from build123d import *

# Parameters (mm, degrees)
BOSS_EXTRUDE1_DEPTH      = 10.6
BOSS_EXTRUDE1_DEPTH_BACK = 26.9
SKETCH1_W                = 40
SKETCH1_H                = 20
SKETCH1_3_W              = 40
SKETCH1_3_H              = 20
SKETCH1_3_W_2            = 7
SKETCH1_3_R              = 2
BOSS_EXTRUDE2_DEPTH      = 3
SKETCH2_R                = 3.307057182
BOSS_EXTRUDE3_DEPTH      = 1.5
BOSS_EXTRUDE4_START      = 1.5
SKETCH2_3_R              = 5.189986332
SKETCH2_3_R_2            = 3.307057182
BOSS_EXTRUDE4_DEPTH      = 6.5
FILLET1_R                = 3
FILLET2_R                = 1
BOSS_EXTRUDE6_DEPTH      = 1


with BuildPart() as part:
    # Sketch1 → Boss-Extrude1 (new, two sides: drawn at the far end of the back side and taken through both)
    with BuildSketch(Plane.XY.offset(-BOSS_EXTRUDE1_DEPTH_BACK)):
        Rectangle(SKETCH1_W, SKETCH1_H)
    extrude(amount=BOSS_EXTRUDE1_DEPTH + BOSS_EXTRUDE1_DEPTH_BACK)

    # Sketch1<3> → Boss-Extrude2 (add)
    # profile 1 of 3: a face of its own
    with BuildSketch(Plane.XY):
        Rectangle(SKETCH1_3_W, SKETCH1_3_H)
    # profile 2 of 3: a face of its own
    with BuildSketch(Plane.XY):
        with Locations((-23.5, 0)):
            Rectangle(SKETCH1_3_W_2, SKETCH1_3_H)
        with Locations((-24.3, -4.95)):
            Circle(SKETCH1_3_R, mode=Mode.SUBTRACT)
        with Locations((-24.3, 4.95)):
            Circle(SKETCH1_3_R, mode=Mode.SUBTRACT)
    # profile 3 of 3: a face of its own
    with BuildSketch(Plane.XY):
        with Locations((23.5, 0)):
            Rectangle(SKETCH1_3_W_2, SKETCH1_3_H)
        with Locations((24.3, -4.95)):
            Circle(SKETCH1_3_R, mode=Mode.SUBTRACT)
        with Locations((24.3, 4.95)):
            Circle(SKETCH1_3_R, mode=Mode.SUBTRACT)
    extrude(amount=BOSS_EXTRUDE2_DEPTH)

    # Sketch2 → Boss-Extrude3 (add)
    with BuildSketch(Plane.XY.offset(10.6)):
        with Locations((10, 0)):
            Circle(SKETCH2_R)
    extrude(amount=BOSS_EXTRUDE3_DEPTH)

    # Sketch2<3> → Boss-Extrude4 (add)
    # profile 1 of 2: a face of its own
    with BuildSketch(Plane.XY.offset(10.6).offset(BOSS_EXTRUDE4_START)):
        with Locations(Location((10, 0, 0), (0, 0, 180))):
            Circle(SKETCH2_3_R)
        with Locations((10, 0)):
            Circle(SKETCH2_3_R_2, mode=Mode.SUBTRACT)
    # profile 2 of 2: a face of its own
    with BuildSketch(Plane.XY.offset(10.6).offset(BOSS_EXTRUDE4_START)):
        with Locations((10, 0)):
            Circle(SKETCH2_3_R_2)
    extrude(amount=BOSS_EXTRUDE4_DEPTH)

    # Fillet1
    fillet1_edges = [part.edges().sort_by_distance(p)[0] for p in [
        (-27, 10, 1.5),
        (-27, -10, 1.5),
        (27, -10, 1.5),
        (27, 10, 1.5),
    ]]
    fillet(fillet1_edges, radius=FILLET1_R)

    # Fillet2
    fillet2_edges = [part.edges().sort_by_distance(p)[0] for p in [
        (20, 0, -26.9),
        (0, 10, 10.6),
        (-20, 0, 10.6),
        (0, -10, 10.6),
        (20, 0, 10.6),
        (0, 10, -26.9),
        (-20, 0, -26.9),
        (-20, -10, 6.8),
        (-20, 10, 6.8),
        (20, 10, 6.8),
        (0, -10, -26.9),
        (-20, -10, -13.45),
        (-20, 10, -13.45),
        (20, 10, -13.45),
        (20, -10, -13.45),
    ]]
    fillet(fillet2_edges, radius=FILLET2_R)

    # Sketch4 → Boss-Extrude6 (add, symmetric)
    with BuildSketch(Plane(origin=(0, 0, 0), x_dir=(1, 0, 0), z_dir=(0, 1, 0))):
        Polygon((-27, -3), (-20, -5.826634937), (-20, -3), align=None)
    boss_extrude6 = extrude(amount=BOSS_EXTRUDE6_DEPTH, both=True)

    # Mirror1: Boss-Extrude6 across plane
    add(boss_extrude6.mirror(Plane(origin=(0, 0, 0), x_dir=(0, 0, 1), z_dir=(1, 0, 0))))


solid = part.part
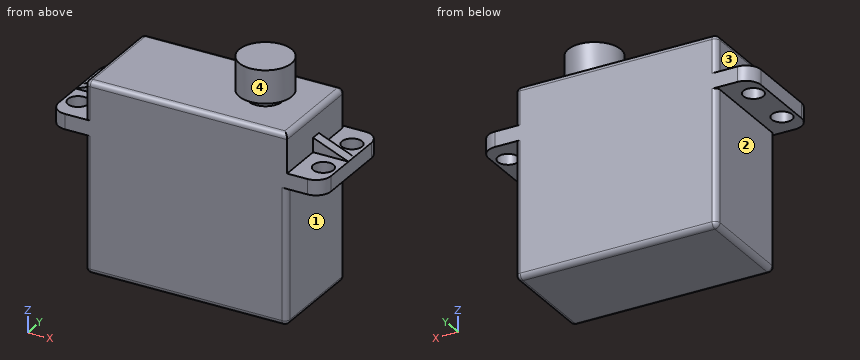
Model file for the job. Use its own axes, mm. Face numbers are marked on the shaded views. A direction names the side the tool comes from. Give positions to 0.01 mm unless a question says otherwise; leave off trailing zeros. Loops run counter-clockwise (first coordinate to the right, second up) from the corner with the lowest first, then second, coordinate; pieces in that order, holes last. Notation, with made-up numbers: (38.25, 68.5) - (75.25, 68.5) arc R24 ccw to (75.25, 102.5) - close; hole circle Ø5 at (30, 18). An arc over 180 degrees is marked (long way). Use one line per item in the form item = value.
(1) Drop flat-ended pins along their axis: P1, Ø3, axis at y = 6, z = -10, coming from the +X side; P2, Ø1, axis at x = 21, y = 8, coming from the -Z side; P3, Ø2.5, axis at x = 24, y = 6, coming from the +Z side. Give the stop position or say it passes through.
Determined:
P1 = 20
P2 = 0
P3 = 3
(2) Drill centre lines: L1, parallel to Y at x = 24.3, z = 1; L2, parallel to Z at x = 3, y = 7.5; L3, parallel to X at y = -6, z = -8. Where is each one in solid material? Low to high.
Determined:
L1 = -9.98 to -6.95, -2.95 to 2.95, 6.95 to 9.98
L2 = -26.9 to 10.6
L3 = -20 to 20
(3) Cut at B-B (z = -18.5). Give the cut face in (x, y), then the cut area to 3 significant figures.
Determined:
outline = (-20, -9) arc R1 ccw to (-19, -10) - (19, -10) arc R1 ccw to (20, -9) - (20, 9) arc R1 ccw to (19, 10) - (-19, 10) arc R1 ccw to (-20, 9) - close
area = 799 mm^2
(4) 3-axis set-ups, long thin cutter, end or side, ignore diameter. For the marked faces 1, 2, 3 and 4: which of +Z, -Z, +X, -X, +Y, -Y reach the whole face in a straight line?
Determined:
face_1 = -Z, +X, +Y, -Y
face_2 = -Z, -X, +Y, -Y
face_3 = +Z, -X
face_4 = +Z
(5) Cut at D-D (y = -4). Give the cut face in (x, z), then the cut area to 3 significant figures.
Determined:
outline = (-27, 0) - (-26.06, 0) - (-26.06, 3) - (-27, 3) - close; (-22.54, 0) - (-20, 0) - (-20, -25.9) arc R1 ccw to (-19, -26.9) - (19, -26.9) arc R1 ccw to (20, -25.9) - (20, 0) - (22.54, 0) - (22.54, 3) - (20, 3) - (20, 9.6) arc R1 ccw to (19, 10.6) - (-19, 10.6) arc R1 ccw to (-20, 9.6) - (-20, 3) - (-22.54, 3) - close; (6.69, 12.1) - (13.31, 12.1) - (13.31, 18.6) - (6.69, 18.6) - close; (26.06, 0) - (27, 0) - (27, 3) - (26.06, 3) - close
area = 1,560 mm^2
(6) Cut at C-C (y = 0). Give the cut face in (x, z).
Determined:
outline = (-27, 0) - (-20, 0) - (-20, -25.9) arc R1 ccw to (-19, -26.9) - (19, -26.9) arc R1 ccw to (20, -25.9) - (20, 0) - (27, 0) - (27, 3) - (20, 5.83) - (20, 9.6) arc R1 ccw to (19, 10.6) - (13.31, 10.6) - (13.31, 12.1) - (15.19, 12.1) - (15.19, 18.6) - (4.81, 18.6) - (4.81, 12.1) - (6.69, 12.1) - (6.69, 10.6) - (-19, 10.6) arc R1 ccw to (-20, 9.6) - (-20, 5.83) - (-27, 3) - close
(7) Cut at A-A (x = -9). Give the cut face in (y, z), then the cut area to 3 significant figures.
Determined:
outline = (-10, -25.9) arc R1 ccw to (-9, -26.9) - (9, -26.9) arc R1 ccw to (10, -25.9) - (10, 9.6) arc R1 ccw to (9, 10.6) - (-9, 10.6) arc R1 ccw to (-10, 9.6) - close
area = 749 mm^2
